Geometry: final body of the model. Coordinates: model frame, mm. Face numbers are marked on the shaded views. Give positions to 0.01 mm unless a question says otherwise; leave off trailing zeros. Write each loop counter-clockwise with the first axis right and the second up, starting at its lowest first coordinate (ties: lowest second). Pieces come first, ordered by that corner, then holes. Notation, with made-up numbers: (63, -33) -> (67, -33) arc R32 cw to (67, -6) -> close; hole circle Ø2 at (68, -29). An arc over 180 degrees is marked (long way). Answer as a JSON object with one key per item and string values.
from build123d import *

# Parameters (mm, degrees)
SKETCH1_R           = 0.85
BOSS_EXTRUDE1_DEPTH = 1


with BuildPart() as part:
    # Sketch1 → Boss-Extrude1 (new body)
    with BuildSketch(Plane(origin=(0, 0, -0.5), x_dir=(-1, 0, 0), z_dir=(0, 0, -1))):
        with BuildLine():
            Line((-3.2, -6.138229217), (-3.2, -7.435859975))
            ThreePointArc((-3.2, -7.435859975), (-3.002328658, -8.03274248), (-2.487462552, -8.393651853))
            Line((-2.487462552, -8.393651853), (-1.286310177, -8.754154311))
            ThreePointArc((-1.286310177, -8.754154311), (-1.144119993, -8.785754135), (-0.998847625, -8.796362433))
            Line((-0.998847625, -8.796362433), (-0.2, -8.796362433))
            Line((-0.2, -8.796362433), (-0.2, -5.496362433))
            ThreePointArc((-0.2, -5.496362433), (0, 5.5), (0.2, -5.496362433))
            Line((0.2, -5.496362433), (0.2, -8.796362433))
            Line((0.2, -8.796362433), (0.998847625, -8.796362433))
            ThreePointArc((0.998847625, -8.796362433), (1.144119993, -8.785754135), (1.286310177, -8.754154311))
            Line((1.286310177, -8.754154311), (2.487462552, -8.393651853))
            ThreePointArc((2.487462552, -8.393651853), (3.002328658, -8.03274248), (3.2, -7.435859975))
            Line((3.2, -7.435859975), (3.2, -6.138229217))
            ThreePointArc((3.2, -6.138229217), (3.262706314, -5.895795241), (3.43509693, -5.71416983))
            ThreePointArc((3.43509693, -5.71416983), (5.631574679, -3.736271631), (7.018174039, -1.125919546))
            ThreePointArc((7.018174039, -1.125919546), (7.251184268, 0.087807561), (7.179369434, 1.32161058))
            ThreePointArc((7.179369434, 1.32161058), (0, 7.3), (-7.179369434, 1.32161058))
            ThreePointArc((-7.179369434, 1.32161058), (-7.251184268, 0.087807561), (-7.018174039, -1.125919546))
            ThreePointArc((-7.018174039, -1.125919546), (-5.631574679, -3.736271631), (-3.43509693, -5.71416983))
            ThreePointArc((-3.43509693, -5.71416983), (-3.262706314, -5.895795241), (-3.2, -6.138229217))
        make_face()
        with Locations((-1.5, -7.296362433)):
            Circle(SKETCH1_R, mode=Mode.SUBTRACT)
        with Locations((1.5, -7.296362433)):
            Circle(SKETCH1_R, mode=Mode.SUBTRACT)
    extrude(amount=-BOSS_EXTRUDE1_DEPTH)


solid = part.part
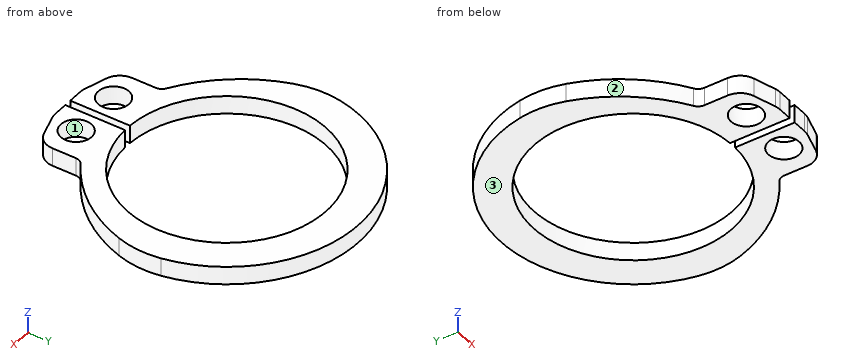
Q1. Cut plane A-A (x = -1.5). Return the cut outline in (y, z).
Values:
{"outline": "(-8.69, -0.5) -> (-8.15, -0.5) -> (-8.15, 0.5) -> (-8.69, 0.5) -> close; (-6.45, -0.5) -> (-5.29, -0.5) -> (-5.29, 0.5) -> (-6.45, 0.5) -> close; (5.29, -0.5) -> (7.14, -0.5) -> (7.14, 0.5) -> (5.29, 0.5) -> close"}
Q2. Cut plane B-B (y = -3.75). Return the cut outline in (x, z).
Values:
{"outline": "(-5.62, -0.5) -> (-4.02, -0.5) -> (-4.02, 0.5) -> (-5.62, 0.5) -> close; (4.02, -0.5) -> (5.62, -0.5) -> (5.62, 0.5) -> (4.02, 0.5) -> close"}
Q3. Material intervals for L1, parallel to X at y = -7.75, z = -0.1; L2, parallel to Y at x = 2, z = 0.2; L3, parallel to Y at x = 1.5, z = 0.2, sorted ascending. Write a range as from..to.
Values:
{"L1": "-3.15..-2.22, -0.78..-0.2, 0.2..0.78, 2.22..3.15", "L2": "-8.54..-7.98, -6.61..-5.12, 5.12..7.02", "L3": "-8.69..-8.15, -6.45..-5.29, 5.29..7.14"}
Q4. Mould query, pull axis X, two halves, no side actions, for the marked faces 1, 2 and 3. Classes: pulls with the +X half, pulls with the -X half, needs draft (parallel to the pull), parting line crosses it, or undercut.
Values:
{"face 1": "undercut", "face 2": "pulls with the -X half", "face 3": "needs draft"}
Q5. First-contact query: P1, Ø4, axis at x = 3.5, y = 2.5, coming from the -Z side. Flat tip, straight axial feed; report the tip coordinate or a pass-through.
Values:
{"P1": "z = -0.5"}
Q6. Cut plane D-D (z = 0.05). Return the cut outline in (x, y), and give its area (3 significant figures).
Values:
{"outline": "(-7.18, 1.32) arc R5 ccw to (-7.02, -1.13) arc R8.5 ccw to (-3.44, -5.71) arc R0.5 cw to (-3.2, -6.14) -> (-3.2, -7.44) arc R1 ccw to (-2.49, -8.39) -> (-1.29, -8.75) arc R1 ccw to (-1, -8.8) -> (-0.2, -8.8) -> (-0.2, -5.5) arc R5.5 cw (long way) to (0.2, -5.5) -> (0.2, -8.8) -> (1, -8.8) arc R1 ccw to (1.29, -8.75) -> (2.49, -8.39) arc R1 ccw to (3.2, -7.44) -> (3.2, -6.14) arc R0.5 cw to (3.44, -5.71) arc R8.5 ccw to (7.02, -1.13) arc R5 ccw to (7.18, 1.32) arc R7.3 ccw to start; hole circle Ø1.7 at (-1.5, -7.3); hole circle Ø1.7 at (1.5, -7.3)", "area": "69.2 mm²"}
Q7. Cut plane C-C (x = -5.25). Return the cut outline in (y, z), and give its area (3 significant figures).
Values:
{"outline": "(-4.19, -0.5) -> (-1.64, -0.5) -> (-1.64, 0.5) -> (-4.19, 0.5) -> close; (1.64, -0.5) -> (5.07, -0.5) -> (5.07, 0.5) -> (1.64, 0.5) -> close", "area": "5.98 mm²"}
